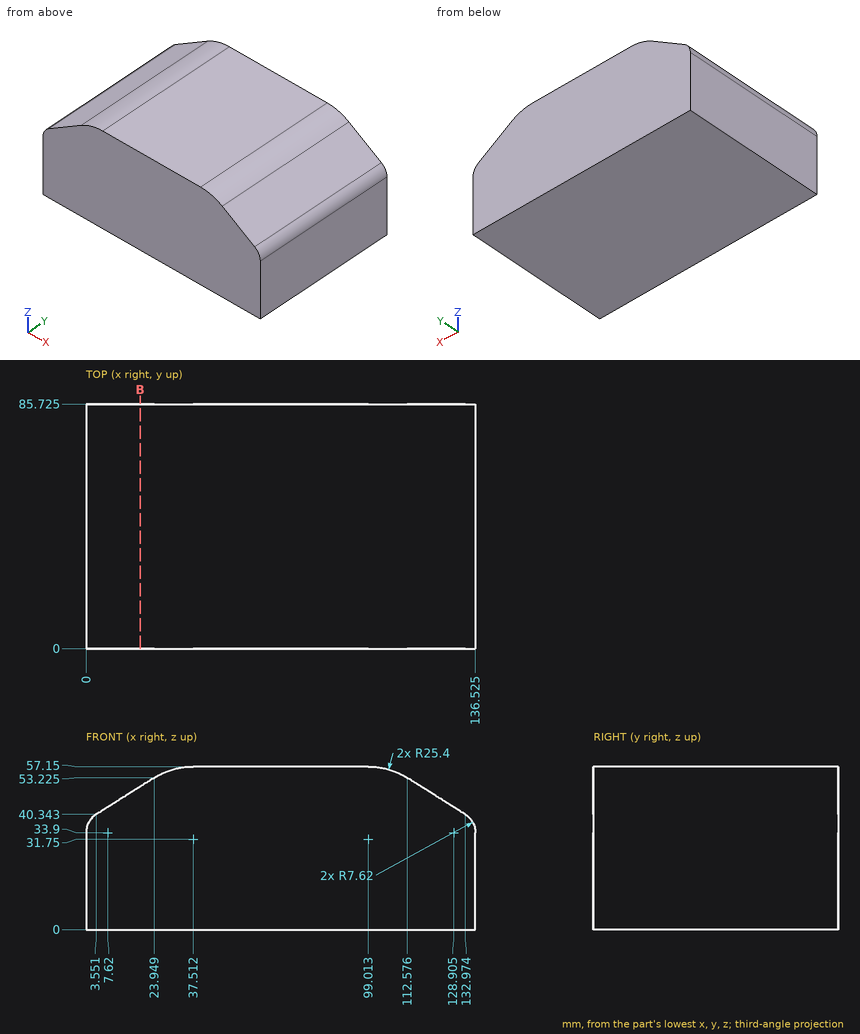
Design review of the part shown in the three views and the two pictorial views. Dimensions are in mm from the part's minimum x, y and z. Coordinates: 2 decimals unless noted, no trailing zeros. Write each loop counter-clockwise with the first axis right and the second up, starting at its lowest first coordinate (ties: lowest second). Pieces come first, ordered by that corner, then holes.
(1) Add section B-B on x = 19. Give the boundary of the cut face in (y, z) (1 decimal), then the cut area to 4 significant figures.
(2) For pin 1 Ø3 at (y, z) = (38, 47.5) entering from +X (1 decimal); pin 2 Ø5 at (x, y) = (26.5, 33) entering from +Z, all flat-tipped, find the tip position at first contact; note any pin that passes through.
(3) Wall thickness on probe 1 along Z at (x, y) = (24, 78); probe 2 along Z at (x, y) = (112, 41.5); probe 3 along X at (y, z) = (53, 36) (1 decimal): over which ranges is each line inside the solid? List them lowest first.
Answer sheet:
1. outline: (0, 0) - (85.7, 0) - (85.7, 50.1) - (0, 50.1) - close
1. area: 4,295 mm2
2. pin 1: stops at x = 124
2. pin 2: stops at z = 55.68
3. probe 1: z = 0 to 53.26
3. probe 2: z = 0 to 53.58
3. probe 3: x = 0.3 to 136.2
